Here's how the part is built. I have some questions about the finished solid (model axes, mm). A direction names the side the tool comes from. Coordinates: 2 decimals unless noted, no trailing zeros. Answer as a JSON object with one key per item and string values. Group by question number.
1) Which directions (+Z, -Z, +X, -X, +Y, -Y) give clear straight access to the entire face, cutting with the end or side of a thin tool? Please do faces 4 (the flat face through (7, 191.102, -10)), 5 (the flat face through (7, -186, -7.87)), 6 (the flat face through (15, -40, 5)).
2) I'm going to push flat-ended pins straight in: pin 1 (4 mm diameter, centred on x = 3, z = 11, fed in from +Y); pin 2 (4.5 mm diameter, centred on x = 4, z = 0.5, fed in from -Y); pin 3 (7.5 mm diameter, centred on x = 6, y = -184.5, fed in from +Z); pin 4 (4 mm diameter, centred on x = 12.5, z = 11.5, fed in from +Y). Where does each tip first touch, or does it pass through?
3) I need wall thicknesses on probe 1 along Y at (x, z) = (9.5, -8.5); probe 2 along X at (y, z) = (-114.5, 50.5); probe 3 along Z at (x, y) = (4.25, 59). Which ranges of each line are inside material? Lowest first, please. Write a range as [from, to].
4) If we mould it in two halves opening along Z, with no side actions, what happens to faces 1 (the flat face through (5, -193.898, -19)), 2 (the flat face through (4.93, 9.45, 39.21)), 3 (the flat face through (7, 198, -2.87))? For each: +Z half, -Z half, draft (parallel to the pull), parting line (faces both ways), or undercut.
```python
from build123d import *

# Parameters (mm, degrees)
F1_DEPTH     = 15
F2_R         = 5
F3_T1_DEPTH  = 418.0350652296
F4_T1_DEPTH  = 390
F4_T3_DEPTH  = 22.5
F4_T5_DEPTH  = 21.0347777317
F4_T7_DEPTH  = 24.1597777317
F4_T12_DEPTH = 5
F4_T18_DEPTH = 5
F4_T22_ANGLE = 90
F4_T24_ANGLE = 90
F5_T1_DEPTH  = 415.7168298797


# Not quite as in the source:
# - a fillet or chamfer that OpenCascade refuses, or shapes differently, is made with other operations: its cross-section is extruded or revolved along the edge and cut away or added


with BuildPart() as f1:
    # F0 (on Right) → F1 (new body)
    with BuildSketch(Plane.YZ):
        Polygon((-193.8978725672, -35.3695585671), (206.1021274328, -35.3695585671), (206.1021274328, -17.8695585671), (191.1021274328, -17.8695585671), (191.1021274328, -2.8695585671), (206.1021274328, -2.8695585671), (206.1021274328, 14.6304414329), (-193.8978725672, 64.6304414329), (-193.8978725672, 37.1304414329), (-178.8978725672, 37.1304414329), (-178.8978725672, 22.1304414329), (-193.8978725672, 22.1304414329), (-193.8978725672, 7.1304414329), (-178.8978725672, 7.1304414329), (-178.8978725672, -7.8695585671), (-193.8978725672, -7.8695585671), align=None)
    extrude(amount=F1_DEPTH)

    # F2
    f2_edges = [f1.edges().sort_by_distance(p)[0] for p in [
        (15, 206.102127, 5.880441),
        (15, 206.102127, -26.619559),
        (15, -193.897873, -21.619559),
        (15, -193.897873, 14.630441),
        (15, -193.897873, 50.880441),
    ]]
    fillet(f2_edges, radius=F2_R)

    # F3: fillet of radius 5 on 1 edges, made by hand

    # F3_s2 → F3_t1 (cut)
    with BuildSketch(Plane(origin=(0, 208.5341292164, -26.0667661521), x_dir=(1, 0, 0), z_dir=(0, -0.9922778767, 0.1240347346))):
        with BuildLine():
            ThreePointArc((15, 35.0812860348), (13.5355339059, 38.6168199408), (10, 40.0812860348))
            Line((10, 40.0812860348), (15, 40.0812860348))
            Line((15, 40.0812860348), (15, 35.0812860348))
        make_face()
    extrude(amount=F3_T1_DEPTH, mode=Mode.SUBTRACT)

    # F4: fillet of radius 5 on 7 edges, made by hand

    # F4_s2 → F4_t1 (cut)
    with BuildSketch(Plane.XZ.offset(-201.1021274328)):
        with BuildLine():
            ThreePointArc((15, -30.3695585671), (13.5355339059, -33.905092473), (10, -35.3695585671))
            Line((10, -35.3695585671), (15, -35.3695585671))
            Line((15, -35.3695585671), (15, -30.3695585671))
        make_face()
    extrude(amount=F4_T1_DEPTH, mode=Mode.SUBTRACT)

    # F4_s4 → F4_t3 (cut)
    with BuildSketch(Plane.YZ.offset(-12.5)):
        with BuildLine():
            ThreePointArc((-193.8978725672, -30.3695585671), (-192.4334064731, -33.905092473), (-188.8978725672, -35.3695585671))
            Line((-188.8978725672, -35.3695585671), (-193.8978725672, -35.3695585671))
            Line((-193.8978725672, -35.3695585671), (-193.8978725672, -30.3695585671))
        make_face()
        with BuildLine():
            ThreePointArc((201.1021274328, -35.3695585671), (204.6376613388, -33.905092473), (206.1021274328, -30.3695585671))
            Line((206.1021274328, -30.3695585671), (206.1021274328, -35.3695585671))
            Line((206.1021274328, -35.3695585671), (201.1021274328, -35.3695585671))
        make_face()
    extrude(amount=F4_T3_DEPTH, mode=Mode.SUBTRACT)

    # F4_s6 → F4_t5 (cut)
    with BuildSketch(Plane.YZ.offset(-11.0347777317)):
        with BuildLine():
            ThreePointArc((206.1021274328, 10.2165303402), (204.8505183119, 13.5255431564), (201.7223011058, 15.1779197238))
            Line((201.7223011058, 15.1779197238), (206.1021274328, 14.6304414329))
            Line((206.1021274328, 14.6304414329), (206.1021274328, 10.2165303402))
        make_face()
    extrude(amount=F4_T5_DEPTH, mode=Mode.SUBTRACT)

    # F4_s8 → F4_t7 (cut)
    with BuildSketch(Plane.YZ.offset(-14.1597777317)):
        with BuildLine():
            ThreePointArc((-188.2776988942, 63.9279197238), (-192.2068853834, 62.7149212193), (-193.8978725672, 58.9665303402))
            Line((-193.8978725672, 58.9665303402), (-193.8978725672, 64.6304414329))
            Line((-193.8978725672, 64.6304414329), (-188.2776988942, 63.9279197238))
        make_face()
    extrude(amount=F4_T7_DEPTH, mode=Mode.SUBTRACT)


with BuildPart() as f4_tool10:
    # F4_s11 → F4_t12 (new body)
    with BuildSketch(Plane.YZ.offset(10)):
        Polygon((-188.8978725672, 58.9665303402), (-188.2776988942, 63.9279197238), (-193.8978725672, 64.6304414329), (-193.8978725672, 58.9665303402), align=None)
    extrude(amount=F4_T12_DEPTH)

    # F4_s13 → F4_t14 (revolve, cut)
    with BuildSketch(Plane(origin=(10, -188.8978725672, 58.9665303402), x_dir=(0, 0.6618025632, -0.7496781758), z_dir=(0, -0.7496781758, -0.6618025632))):
        with BuildLine():
            ThreePointArc((0, -5), (5, 0), (0, 5))
            Line((0, 5), (0, -5))
        make_face()
    revolve(axis=Axis((10, -188.8978725672, 58.9665303402), (1, 0, 0)), mode=Mode.SUBTRACT)


with BuildPart() as f1_1:
    add(f1.part)

    # F4_t9: cut F4_tool10
    add(f4_tool10.part, mode=Mode.SUBTRACT)


with BuildPart() as f4_tool16:
    # F4_s17 → F4_t18 (new body)
    with BuildSketch(Plane.YZ.offset(10)):
        Polygon((201.1021274328, 10.2165303402), (206.1021274328, 10.2165303402), (206.1021274328, 14.6304414329), (201.7223011058, 15.1779197238), align=None)
    extrude(amount=F4_T18_DEPTH)

    # F4_s19 → F4_t20 (revolve, cut)
    with BuildSketch(Plane(origin=(10, 201.1021274328, 10.2165303402), x_dir=(0, -0.7496781758, -0.6618025632), z_dir=(0, -0.6618025632, 0.7496781758))):
        with BuildLine():
            ThreePointArc((0, -5), (5, 0), (0, 5))
            Line((0, 5), (0, -5))
        make_face()
    revolve(axis=Axis((10, 201.1021274328, 10.2165303402), (1, 0, 0)), mode=Mode.SUBTRACT)


with BuildPart() as f1_2:
    add(f1_1.part)

    # F4_t15: cut F4_tool16
    add(f4_tool16.part, mode=Mode.SUBTRACT)

    # F4_s21 → F4_t22 (revolve, cut)
    with BuildSketch(Plane.YZ.offset(10)):
        with BuildLine():
            ThreePointArc((-188.8978725672, -35.3695585671), (-192.4334064731, -33.905092473), (-193.8978725672, -30.3695585671))
            Line((-193.8978725672, -30.3695585671), (-193.8978725672, -35.3695585671))
            Line((-193.8978725672, -35.3695585671), (-188.8978725672, -35.3695585671))
        make_face()
    revolve(axis=Axis((10, -188.8978725672, -35.3695585671), (0, 0, 1)), revolution_arc=F4_T22_ANGLE, mode=Mode.SUBTRACT)

    # F4_s23 → F4_t24 (revolve, cut)
    with BuildSketch(Plane.YZ.offset(10)):
        with BuildLine():
            ThreePointArc((201.1021274328, -35.3695585671), (204.6376613388, -33.905092473), (206.1021274328, -30.3695585671))
            Line((206.1021274328, -30.3695585671), (206.1021274328, -35.3695585671))
            Line((206.1021274328, -35.3695585671), (201.1021274328, -35.3695585671))
        make_face()
    revolve(axis=Axis((10, 201.1021274328, -35.3695585671), (0, 0, -1)), revolution_arc=F4_T24_ANGLE, mode=Mode.SUBTRACT)

    # F5: chamfer of 5 on 1 edges, made by hand

    # F5_s2 → F5_t1 (cut)
    with BuildSketch(Plane.XZ.offset(-213.9605423726)):
        Polygon((0, -30.3695585671), (5, -35.3695585671), (0, -35.3695585671), align=None)
    extrude(amount=F5_T1_DEPTH, mode=Mode.SUBTRACT)


solid = f1_2.part
```
Determined:
{
 "1": {"face 4": "+X, -X, +Y", "face 5": "+X, -X, -Y", "face 6": "+Z, -Z, +X, +Y, -Y"},
 "2": {"pin 1": "y = 206.1", "pin 2": "y = -178.9", "pin 3": "z = 63.92", "pin 4": "y = 206.04"},
 "3": {"probe 1": "[-193.9, 191.1]", "probe 2": "[0, 14.93]", "probe 3": "[-34.62, 33.02]"},
 "4": {"face 1": "draft", "face 2": "+Z half", "face 3": "undercut"}
}
